Input: part model. Units: mm. Frame: model coordinates. A direction names the side the tool comes from. Coordinates: 2 decimals unless noted, no trailing zeros. Loops run counter-clockwise (first coordinate to the right, second up) from the corner with the lowest first, then second, coordinate; pieces in that order, holes last.
(1) Contact query for flat-ended pins moving along their axis: P1, Ø1.5, axis at x = -7.5, y = -14, coming from the +Z side; P2, Ø1.5, axis at y = -22, z = -2.5, coming from the -X side. Output: stop coordinate, or through.
(2) Section B-B, the plane y = -34.5. Return loops of the section in (x, z), then the cut area to 3 significant figures.
(3) Section A-A, the plane z = 5.5. Return loops of the section in (x, y).
(4) Set-up query: faces 1 (the face through (0, -30.5, 4)), 2 (the face through (0, 0, -2)), 3 (the face through (0, -21, -4)). Return all of +Z, -Z, +X, -X, +Y, -Y with unobstructed straight access to the full face (end or side cutting, diameter ignored); none if empty.
(5) Section D-D, the plane y = -19. Return loops of the section in (x, z), then the cut area to 3 significant figures.
(6) Mould query, pull axis Z, two halves, no side actions, for faces 4 (the face through (0, -9.5, -2)), 5 (the face through (0, -21, -13)), 6 (the face through (21, -21, -5)). Classes: released by +Z, released by -Z, zero draft, split by the parting line, or undercut.
(7) Section C-C, the plane x = -2. Return loops of the section in (y, z), then the cut area to 3 significant figures.
(8) Line query: L1, parallel to Y at x = -18.5, z = 0.75; L2, parallel to Y at x = 4, z = -1; L3, parallel to Z at x = 8.5, y = -32. Output: solid intervals per line, ascending.
```python
from build123d import *

# Parameters (mm, degrees)
F1_DEPTH = 42
F2_W     = 9.5
F2_H     = 9
F3_DEPTH = 42


with BuildPart() as f1:
    # F0 (on Front) → F1 (new body)
    with BuildSketch(Plane.XZ):
        with BuildLine():
            Line((-21, -13), (-3.5, -13))
            Line((-3.5, -13), (-3.5, -2.5))
            ThreePointArc((-3.5, -2.5), (-6, 0), (-3.5, 2.5))
            Line((-3.5, 2.5), (-3.5, 9))
            Line((-3.5, 9), (-21, 9))
            Line((-21, 9), (-21, -13))
        make_face()
        with BuildLine():
            Line((-3.5, -13), (21, -13))
            Line((21, -13), (21, 9))
            Line((21, 9), (-3.5, 9))
            Line((-3.5, 9), (-3.5, 2.5))
            ThreePointArc((-3.5, 2.5), (-1.732233, 1.767767), (-1, 0))
            ThreePointArc((-1, 0), (-1.732233, -1.767767), (-3.5, -2.5))
            Line((-3.5, -2.5), (-3.5, -13))
        make_face()
    extrude(amount=F1_DEPTH)

    # F2 (on face) → F3 (cut)
    with BuildSketch(Plane.YZ.offset(21)):
        with Locations((-25.75, 4.5)):
            Rectangle(F2_W, F2_H)
        with Locations((-16.25, 4.5)):
            Rectangle(F2_W, F2_H)
        Polygon((-32.5, -4), (-21, -4), (-21, 0), (-30.5, 0), (-32.5, 0), align=None)
        Polygon((-21, 0), (-21, -4), (-9.5, -4), (-9.5, 0), (-11.5, 0), align=None)
    extrude(amount=-F3_DEPTH, mode=Mode.SUBTRACT)


solid = f1.part
```
Report:
1. P1: stops at z = -4
1. P2: passes through
2. outline: (-21, -13) - (21, -13) - (21, 9) - (-21, 9) - close; hole circle Ø5 at (-3.5, 0)
2. area: 904 mm2
3. outline: (-21, -42) - (21, -42) - (21, -30.5) - (-21, -30.5) - close; (-21, -11.5) - (21, -11.5) - (21, 0) - (-21, 0) - close
4. face 1: +Z, +X, -X
4. face 2: +Z, -Z, +X, -X, +Y
4. face 3: +X, -X
5. outline: (-21, -13) - (21, -13) - (21, -4) - (-21, -4) - close
5. area: 378 mm2
6. face 4: undercut
6. face 5: released by -Z
6. face 6: zero draft
7. outline: (-42, -13) - (0, -13) - (0, -2) - (-9.5, -2) - (-9.5, -4) - (-32.5, -4) - (-32.5, -2) - (-42, -2) - close; (-42, 2) - (-30.5, 2) - (-30.5, 9) - (-42, 9) - close; (-11.5, 2) - (0, 2) - (0, 9) - (-11.5, 9) - close
7. area: 577 mm2
8. L1: y = -42 to -30.5, -11.5 to 0
8. L2: y = -42 to -32.5, -9.5 to 0
8. L3: z = -13 to -4, 0 to 9
